The figure shows three views and two pictorial views of one solid part (mm, origin at its lowest corner). Answer the questions. A direction names the side the tool comes from. Give positions to 0.01 mm unless a question says otherwise; leave off trailing zeros. Write each loop counter-clockwise with the first axis right and the second up, starting at its lowest first coordinate (ties: lowest second). Pieces come first, ordered by that corner, then holes. Notation, with made-up numbers: M -9.5,-27 L 43.5,-27 A20 cw 43.5,-20 Z; hole C 84,-17 d5. An arc over 180 degrees is marked long. Return JSON: item names as keys, results as strings.
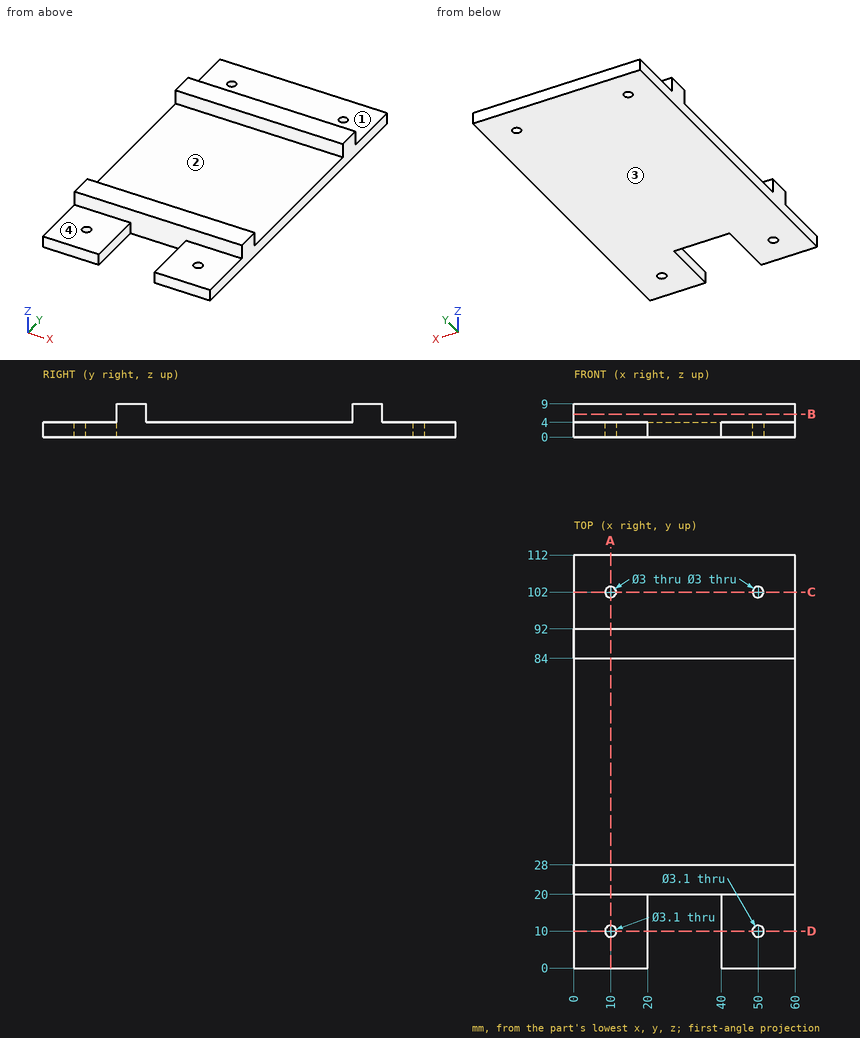
Item 1: A cutting plane is placed at D-D, the plane y = 10. Write down the section's boundary in (x, z), plus the area to 3 significant figures.
Geometry results:
{"outline": "M 0,0 L 8.45,0 L 8.45,4 L 0,4 Z; M 11.55,0 L 20,0 L 20,4 L 11.55,4 Z; M 40,0 L 48.45,0 L 48.45,4 L 40,4 Z; M 51.55,0 L 60,0 L 60,4 L 51.55,4 Z", "area": "135 mm2"}
Item 2: A cutting plane is placed at B-B, the plane z = 6.25. Write down the section's boundary in (x, y).
Geometry results:
{"outline": "M 0,20 L 60,20 L 60,28 L 0,28 Z; M 0,84 L 60,84 L 60,92 L 0,92 Z"}
Item 3: A cutting plane is placed at C-C, the plane y = 102. Write down the section's boundary in (x, z), plus the area to 3 significant figures.
Geometry results:
{"outline": "M 0,0 L 8.5,0 L 8.5,4 L 0,4 Z; M 11.5,0 L 48.5,0 L 48.5,4 L 11.5,4 Z; M 51.5,0 L 60,0 L 60,4 L 51.5,4 Z", "area": "216 mm2"}
Item 4: Which of the six approach directions +Z, -Z, +X, -X, +Y, -Y give full straight-line access (tool end or side, diameter ignored) to the marked faces 3 and 4?
Geometry results:
{"face 3": "-Z, +X, -X, +Y, -Y", "face 4": "+Z, +X, -X, -Y"}
Item 5: Find the intervals of material crossed by line 1 (Y direction, x = 50, z = 1.3); line 2 (X direction, y = 102, z = 1.55); line 3 (Y direction, x = 15, z = 4.5), in increasing order.
Geometry results:
{"line 1": "y = 0 to 8.45, 11.55 to 100.5, 103.5 to 112", "line 2": "x = 0 to 8.5, 11.5 to 48.5, 51.5 to 60", "line 3": "y = 20 to 28, 84 to 92"}
Item 6: A cutting plane is placed at A-A, the plane x = 10. Write down the section's boundary in (y, z), plus the area to 3 significant figures.
Geometry results:
{"outline": "M 0,0 L 8.45,0 L 8.45,4 L 0,4 Z; M 11.55,0 L 100.5,0 L 100.5,4 L 92,4 L 92,9 L 84,9 L 84,4 L 28,4 L 28,9 L 20,9 L 20,4 L 11.55,4 Z; M 103.5,0 L 112,0 L 112,4 L 103.5,4 Z", "area": "504 mm2"}
Item 7: Given pin 1 Ø1 at (x, y) = (39, 57.5) entering from -Z; pin 2 Ø2.5 at (x, y) = (50, 102) entering from +Z; pin 3 Ø17 at (x, y) = (44.5, 42.5) entering from +Z; pin 4 Ø1.5 at (x, z) = (28, 6) entering from +Y, each flat-ended and moving along its own axis, determine where each tip first touches the part or whether it passes through.
Geometry results:
{"pin 1": "stops at z = 0", "pin 2": "passes through", "pin 3": "stops at z = 4", "pin 4": "stops at y = 92"}
Item 8: Determine the mould class of the marked faces 1 and 2 for opening direction Y: +Y half, -Y half, draft (parallel to the pull), parting line (faces both ways), or undercut.
Geometry results:
{"face 1": "draft", "face 2": "undercut"}
